```python
from build123d import *

# Parameters (mm, degrees)
SKIZZE1_R                       = 5
SKIZZE1_R_2                     = 4
AUFSATZ_LINEAR_AUSTRAGEN1_DEPTH = 35
VERRUNDUNG1_R                   = 0.2


with BuildPart() as part:
    # Skizze1 → Aufsatz-Linear austragen1 (new body)
    with BuildSketch(Plane.XY):
        Circle(SKIZZE1_R)
        Circle(SKIZZE1_R_2, mode=Mode.SUBTRACT)
    extrude(amount=AUFSATZ_LINEAR_AUSTRAGEN1_DEPTH)

    # Verrundung1
    verrundung1_edges = [part.edges().sort_by_distance(p)[0] for p in [
        (-5, 0, 0),
        (-5, 0, 35),
        (-4, 0, 0),
        (-4, 0, 35),
    ]]
    fillet(verrundung1_edges, radius=VERRUNDUNG1_R)


solid = part.part
```
Source: CAD feature listing. Evaluate the final solid. Frame: model axes, mm. Give positions to 0.01 mm unless a question says otherwise; leave off trailing zeros. Write each loop counter-clockwise with the first axis right and the second up, starting at its lowest first coordinate (ties: lowest second). Pieces come first, ordered by that corner, then holes.
1. Material intervals for line 1 along Y through (x, z) = (0, 9.5); line 2 along Y through (x, z) = (-1.25, 7.5); line 3 along Z through (x, y) = (4.75, 1), sorted ascending.
2. Section query C-C (z = 10). Return the cut outline in (x, y), then the cut area to 3 significant figures.
3. First-contact query: pin 1 (3 mm diameter, centred on y = 2.5, z = 13, fed in from -X); pin 2 (4 mm diameter, centred on y = -2.5, z = 4.5, fed in from +X). Flat tips, straight axial feed; report the tip coordinate or a pass-through.
4. Pull-direction query (X, two-part tool) for faces 1 (the face through (-1.08, -4.88, 17.26)), 2 (the face through (-0.867, -3.905, 17.258)), 3 (the face through (2, -4, 35)); classes: +X half, -X half, draft (parallel to the pull), parting line (faces both ways), or undercut.
5. Section query A-A (x = 0). Return the cut outline in (y, z), then the cut area to 3 significant figures.
Output values:
1. line 1: y = -5 to -4, 4 to 5
1. line 2: y = -4.84 to -3.8, 3.8 to 4.84
1. line 3: z = 0.01 to 34.99
2. outline: circle Ø10 at (0, 0); hole circle Ø8 at (0, 0)
2. area: 28.3 mm2
3. pin 1: stops at x = -4.9
3. pin 2: stops at x = 4.97
4. face 1: parting line
4. face 2: undercut
4. face 3: draft
5. outline: (-5, 0.2) arc R0.2 ccw to (-4.8, 0) - (-4.2, 0) arc R0.2 ccw to (-4, 0.2) - (-4, 34.8) arc R0.2 ccw to (-4.2, 35) - (-4.8, 35) arc R0.2 ccw to (-5, 34.8) - close; (4, 0.2) arc R0.2 ccw to (4.2, 0) - (4.8, 0) arc R0.2 ccw to (5, 0.2) - (5, 34.8) arc R0.2 ccw to (4.8, 35) - (4.2, 35) arc R0.2 ccw to (4, 34.8) - close
5. area: 69.9 mm2
